```python
from build123d import *
from build123d.topology import SkipClean

# Parameters (mm, degrees)
SKETCH1_W               = 29
SKETCH1_H               = 50
BOSS_EXTRUDE1_DEPTH     = 2.5
SKETCH2_R               = 14.5
SKETCH2_R_2             = 13.8
BOSS_EXTRUDE3_DEPTH     = 6
BOSS_EXTRUDE4_DEPTH     = 6
CUT_EXTRUDE1_DEPTH      = 6
SKETCH5_R               = 0.6
CUT_EXTRUDE2_DEPTH      = 6
CUT_EXTRUDE3_DEPTH      = 10
CUT_EXTRUDE3_DEPTH_BACK = 4
SKETCH6_R               = 1.6
BOSS_EXTRUDE6_DEPTH     = 4
CUT_EXTRUDE4_START      = -8
CUT_EXTRUDE4_DEPTH      = 8
CUT_EXTRUDE5_DEPTH      = 5
SKETCH10_W              = 4.15
SKETCH10_H              = 4.15
SKETCH10_R              = 12.5
CUT_EXTRUDE7_DEPTH      = 1
SKETCH11_W              = 4.15
SKETCH11_H              = 4.15
BOSS_EXTRUDE7_DEPTH     = 2
SKETCH13_R              = 1.1
CUT_EXTRUDE8_DEPTH      = 1.1
SKETCH14_R              = 12.5
CUT_EXTRUDE9_DEPTH      = 1
SKETCH15_R              = 13.8
BOSS_EXTRUDE8_DEPTH     = 0.5
SKETCH16_R              = 14.5
SKETCH16_R_2            = 13.8
BOSS_EXTRUDE9_DEPTH     = 0.5


with BuildPart() as part:
    # Sketch1 → Boss-Extrude1 (new body)
    with BuildSketch(Plane(origin=(0, 0, 0), x_dir=(1, 0, 0), z_dir=(0, 1, 0))):
        with Locations((-98.70287726, -30.536357795)):
            Rectangle(SKETCH1_W, SKETCH1_H)
    extrude(amount=BOSS_EXTRUDE1_DEPTH)

    # Sketch2 → Boss-Extrude3 (add)
    with BuildSketch(Plane(origin=(0, 2.5, 0), x_dir=(1, 0, 0), z_dir=(0, 1, 0))):
        with Locations(Location((-98.70287726, -41.036357795, 0), (0, 0, 270))):
            Circle(SKETCH2_R)
        with Locations(Location((-98.70287726, -41.036357795, 0), (0, 0, 270))):
            Circle(SKETCH2_R_2, mode=Mode.SUBTRACT)
    extrude(amount=BOSS_EXTRUDE3_DEPTH)

    # Sketch3 → Boss-Extrude4 (add)
    with BuildSketch(Plane(origin=(0, 2.5, 0), x_dir=(1, 0, 0), z_dir=(0, 1, 0))):
        with BuildLine():
            Line((-100.672014126, -40.686357795), (-98.70287726, -40.686357795))
            Line((-98.70287726, -40.686357795), (-96.733740393, -40.686357795))
            ThreePointArc((-96.733740393, -40.686357795), (-98.70287726, -39.036357795), (-100.672014126, -40.686357795))
        make_face()
        with BuildLine():
            Line((-96.733740393, -41.386357795), (-100.672014126, -41.386357795))
            ThreePointArc((-100.672014126, -41.386357795), (-98.70287726, -43.036357795), (-96.733740393, -41.386357795))
        make_face()
    extrude(amount=BOSS_EXTRUDE4_DEPTH)

    # Sketch4 → Cut-Extrude1 (cut)
    with BuildSketch(Plane(origin=(0, 2.5, 0), x_dir=(1, 0, 0), z_dir=(0, 1, 0))):
        Polygon((-93.70287726, -26.248512358), (-93.70287726, -14.248512358), (-97.70287726, -14.248512358), (-97.70287726, -20.248512358), (-97.70287726, -26.248512358), align=None)
    extrude(amount=-CUT_EXTRUDE1_DEPTH, mode=Mode.SUBTRACT)

    # Sketch5 → Cut-Extrude2 (cut)
    with BuildSketch(Plane(origin=(0, 0, 26.248512358), x_dir=(-1, 0, 0), z_dir=(0, 0, -1))):
        with Locations((95.70287726, 6)):
            Circle(SKETCH5_R)
    extrude(amount=-CUT_EXTRUDE2_DEPTH, mode=Mode.SUBTRACT)

    # Sketch6 → Cut-Extrude3 (cut, two sides: drawn at the far end of the back side and taken through both)
    with BuildSketch(Plane(origin=(-97.70287726, 0, 0), x_dir=(0, 0, -1), z_dir=(1, 0, 0)).offset(-CUT_EXTRUDE3_DEPTH_BACK)):
        with Locations((-20.248512358, 2.5)):
            Circle(SKETCH6_R)
    extrude(amount=CUT_EXTRUDE3_DEPTH + CUT_EXTRUDE3_DEPTH_BACK, mode=Mode.SUBTRACT)

    # Sketch7 → Boss-Extrude6 (add)
    with SkipClean():  # the faces are left unmerged after this step: merging them gives an invalid solid
        with BuildSketch(Plane(origin=(-97.70287726, 0, 0), x_dir=(0, 0, -1), z_dir=(1, 0, 0))):
            with BuildLine():
                Line((-22.748512358, 2.5), (-21.848512358, 2.5))
                ThreePointArc((-21.848512358, 2.5), (-20.248512358, 4.1), (-18.648512358, 2.5))
                Line((-18.648512358, 2.5), (-17.748512358, 2.5))
                ThreePointArc((-17.748512358, 2.5), (-20.248512358, 5), (-22.748512358, 2.5))
            make_face()
            with BuildLine():
                ThreePointArc((-18.648512358, 2.5), (-20.248512358, 0.9), (-21.848512358, 2.5))
                Line((-21.848512358, 2.5), (-22.748512358, 2.5))
                ThreePointArc((-22.748512358, 2.5), (-20.248512358, 0), (-17.748512358, 2.5))
                Line((-17.748512358, 2.5), (-18.648512358, 2.5))
            make_face()
        extrude(amount=-BOSS_EXTRUDE6_DEPTH)

    # Sketch8 → Cut-Extrude4 (cut)
    with SkipClean():  # the faces are left unmerged after this step: merging them gives an invalid solid
        with BuildSketch(Plane.ZY.offset(93.70287726).offset(CUT_EXTRUDE4_START)):
            with BuildLine():
                Line((20.248512358, 2.5), (18.648512358, 2.5))
                ThreePointArc((18.648512358, 2.5), (19.117141508, 1.36862915), (20.248512358, 0.9))
                Line((20.248512358, 0.9), (20.248512358, 2.5))
            make_face()
            with BuildLine():
                Line((21.848512358, 2.5), (20.248512358, 2.5))
                Line((20.248512358, 2.5), (20.248512358, 0.9))
                ThreePointArc((20.248512358, 0.9), (21.379883208, 1.36862915), (21.848512358, 2.5))
            make_face()
            with BuildLine():
                ThreePointArc((20.248512358, 0.9), (19.117141508, 1.36862915), (18.648512358, 2.5))
                Line((18.648512358, 2.5), (18.648512358, 0.9))
                Line((18.648512358, 0.9), (20.248512358, 0.9))
            make_face()
            with BuildLine():
                ThreePointArc((21.848512358, 2.5), (21.379883208, 1.36862915), (20.248512358, 0.9))
                Line((20.248512358, 0.9), (21.848512358, 0.9))
                Line((21.848512358, 0.9), (21.848512358, 2.5))
            make_face()
        extrude(amount=CUT_EXTRUDE4_DEPTH, mode=Mode.SUBTRACT)

    # Sketch9 → Cut-Extrude5 (cut)
    with SkipClean():  # the faces are left unmerged after this step: merging them gives an invalid solid
        with BuildSketch(Plane(origin=(0, 2.5, 0), x_dir=(1, 0, 0), z_dir=(0, 1, 0))):
            Polygon((-113.20287726, -5.536357795), (-113.20287726, -16.036357795), (-97.70287726, -16.036357795), (-97.70287726, -14.248512358), (-93.70287726, -14.248512358), (-93.70287726, -16.036357795), (-84.20287726, -16.036357795), (-84.20287726, -5.536357795), align=None)
        extrude(amount=-CUT_EXTRUDE5_DEPTH, mode=Mode.SUBTRACT)

    # Sketch10 → Cut-Extrude7 (cut)
    with SkipClean():  # the faces are left unmerged after this step: merging them gives an invalid solid
        with BuildSketch(Plane.XZ):
            with Locations((-111.12787726, 18.111357795)):
                Rectangle(SKETCH10_W, SKETCH10_H)
            with Locations((-86.27787726, 18.111357795)):
                Rectangle(SKETCH10_W, SKETCH10_H)
            with Locations((-111.12787726, 53.461357795)):
                Rectangle(SKETCH10_W, SKETCH10_H)
            with Locations((-86.27787726, 53.461357795)):
                Rectangle(SKETCH10_W, SKETCH10_H)
            with Locations(Location((-98.70287726, 41.036357795, 0), (0, 0, 270))):
                Circle(SKETCH10_R)
        extrude(amount=-CUT_EXTRUDE7_DEPTH, mode=Mode.SUBTRACT)

    # Sketch11 → Boss-Extrude7 (add)
    with SkipClean():  # the faces are left unmerged after this step: merging them gives an invalid solid
        with BuildSketch(Plane(origin=(0, 2.5, 0), x_dir=(1, 0, 0), z_dir=(0, 1, 0))):
            with Locations((-111.12787726, -53.461357795)):
                Rectangle(SKETCH11_W, SKETCH11_H)
            with Locations((-86.27787726, -53.461357795)):
                Rectangle(SKETCH11_W, SKETCH11_H)
            with Locations((-111.12787726, -18.111357795)):
                Rectangle(SKETCH11_W, SKETCH11_H)
            Polygon((-88.35287726, -16.036357795), (-88.35287726, -18.648512358), (-85.70287726, -18.648512358), (-85.70287726, -20.186357795), (-84.20287726, -20.186357795), (-84.20287726, -16.036357795), align=None)
        extrude(amount=BOSS_EXTRUDE7_DEPTH)

    # Sketch13 → Cut-Extrude8 (cut)
    with SkipClean():  # the faces are left unmerged after this step: merging them gives an invalid solid
        with BuildSketch(Plane.XZ.offset(-1)):
            with Locations(Location((-111.12787726, 53.461357795, 0), (0, 0, 270))):
                Circle(SKETCH13_R)
            with Locations(Location((-86.27787726, 53.461357795, 0), (0, 0, 270))):
                Circle(SKETCH13_R)
            with Locations(Location((-111.12787726, 18.111357795, 0), (0, 0, 270))):
                Circle(SKETCH13_R)
            with Locations((-86.27787726, 18.111357795)):
                Circle(SKETCH13_R)
        extrude(amount=-CUT_EXTRUDE8_DEPTH, mode=Mode.SUBTRACT)

    # Sketch14 → Cut-Extrude9 (cut)
    with SkipClean():  # the faces are left unmerged after this step: merging them gives an invalid solid
        with BuildSketch(Plane.XZ.offset(-1)):
            with Locations(Location((-98.70287726, 41.036357795, 0), (0, 0, 270))):
                Circle(SKETCH14_R)
        extrude(amount=-CUT_EXTRUDE9_DEPTH, mode=Mode.SUBTRACT)

    # Sketch15 → Boss-Extrude8 (add)
    with SkipClean():  # the faces are left unmerged after this step: merging them gives an invalid solid
        with BuildSketch(Plane(origin=(0, 2.5, 0), x_dir=(1, 0, 0), z_dir=(0, 1, 0))):
            with Locations(Location((-98.70287726, -41.036357795, 0), (0, 0, 270))):
                Circle(SKETCH15_R)
        extrude(amount=BOSS_EXTRUDE8_DEPTH)

    # Sketch16 → Boss-Extrude9 (add)
    # profile 1 of 3: a face of its own
    with SkipClean():  # the faces are left unmerged after this step: merging them gives an invalid solid
        with BuildSketch(Plane(origin=(0, 8.5, 0), x_dir=(1, 0, 0), z_dir=(0, 1, 0))):
            with Locations(Location((-98.70287726, -41.036357795, 0), (0, 0, 270))):
                Circle(SKETCH16_R)
            with Locations(Location((-98.70287726, -41.036357795, 0), (0, 0, 270))):
                Circle(SKETCH16_R_2, mode=Mode.SUBTRACT)
        # profile 2 of 3: a face of its own
        with BuildSketch(Plane(origin=(0, 8.5, 0), x_dir=(1, 0, 0), z_dir=(0, 1, 0))):
            with BuildLine():
                ThreePointArc((-96.733740393, -40.686357795), (-98.70287726, -39.036357795), (-100.672014126, -40.686357795))
                Line((-100.672014126, -40.686357795), (-96.733740393, -40.686357795))
            make_face()
        # profile 3 of 3: a face of its own
        with BuildSketch(Plane(origin=(0, 8.5, 0), x_dir=(1, 0, 0), z_dir=(0, 1, 0))):
            with BuildLine():
                ThreePointArc((-100.672014126, -41.386357795), (-98.70287726, -43.036357795), (-96.733740393, -41.386357795))
                Line((-96.733740393, -41.386357795), (-100.672014126, -41.386357795))
            make_face()
        extrude(amount=BOSS_EXTRUDE9_DEPTH)


solid = part.part
```
The model under review builds one solid part; all positions refer to its coordinate system, in mm. A direction names the side the tool comes from. Round coordinates to 2 decimals unless told otherwise and drop trailing zeros. Loops run counter-clockwise (first coordinate to the right, second up) from the corner with the lowest first, then second, coordinate; pieces in that order, holes last. Notation, with made-up numbers: (9, -22.5) -> (61, -22.5) arc R35 ccw to (61, 12.5) -> close; hole circle Ø3 at (18, -23.75). An arc over 180 degrees is marked (long way). Answer in a Markdown table with one row per item.
1) Tool access review of faces 1 (the cylindrical face through (-98.742, 5.958, 43.036)), 2 (the flat face through (-86, 4.5, 18)), 3 (the flat face through (-111, 3, 51.386)), 4 (the cylindrical face through (-86.035, 1.542, 17.038)): name each direction out of +Z, -Z, +X, -X, +Y, -Y from which nothing blocks a thin tool from reaching the whole face with its end or side.
Taken from the geometry:
| item | result |
|---|---|
| face 1 | +Y |
| face 2 | -Z, +X, +Y |
| face 3 | -X, +Y |
| face 4 | -Y |
2) For pin 1 Ø2 at (x, y) = (-95, 1.5) entering from -Z; pin 2 Ø2 at (x, z) = (-111.13, 53.46) entering from -Y; pin 3 Ø3 at (x, y) = (-91.5, 4.5) entering from -Z, all flat-tipped, find the tip position at first contact; note any pin that passes through.
Taken from the geometry:
| item | result |
|---|---|
| pin 1 | stops at z = 26.25 |
| pin 2 | stops at y = 2.1 |
| pin 3 | stops at z = 27.7 |
3) Consider section D-D, the plane z = 47. Write out the cut boundary in (x, y), plus the area to 3 significant figures.
Taken from the geometry:
| item | result |
|---|---|
| outline | (-113.2, 0) -> (-109.69, 0) -> (-109.69, 2) -> (-87.72, 2) -> (-87.72, 0) -> (-84.2, 0) -> (-84.2, 2.5) -> (-85.49, 2.5) -> (-85.49, 9) -> (-86.26, 9) -> (-86.26, 3) -> (-111.15, 3) -> (-111.15, 9) -> (-111.92, 9) -> (-111.92, 2.5) -> (-113.2, 2.5) -> close |
| area | 51.0 mm² |
4) Wall thickness on line 1 along Z through (x, y) = (-109.75, 3.75); line 2 along X through (y, z) = (7.75, 40); line 3 along X through (y, z) = (8, 40.5): over which ranges is each line inside the solid? List them lowest first.
Taken from the geometry:
| item | result |
|---|---|
| line 1 | z = 16.04 to 20.19, 31.64 to 32.77, 49.31 to 50.43, 51.39 to 55.54 |
| line 2 | x = -113.17 to -112.46, -100.41 to -96.99, -84.94 to -84.24 |
| line 3 | x = -113.19 to -112.49, -100.63 to -96.78, -84.91 to -84.21 |
5) Consider section C-C, the plane y = 6. Write out the cut boundary in (x, z), plus the area to 3 significant figures.
Taken from the geometry:
| item | result |
|---|---|
| outline | (-100.67, 40.69) arc R2 ccw to (-96.73, 40.69) -> close; (-100.67, 41.39) -> (-96.73, 41.39) arc R2 ccw to start; (-96.3, 26.74) -> (-96.3, 27.45) arc R13.8 cw (long way) to (-95.1, 27.71) -> (-95.1, 26.99) arc R14.5 ccw (long way) to start |
| area | 71.2 mm² |
6) Consider section B-B, the plane y = 8.5. Write out the cut boundary in (x, z).
Taken from the geometry:
| item | result |
|---|---|
| outline | circle Ø29 at (-98.7, 41.04); (-100.67, 40.69) arc R2 ccw to (-96.73, 40.69) -> close; (-100.67, 41.39) -> (-96.73, 41.39) arc R2 ccw to start; hole circle Ø27.6 at (-98.7, 41.04) |
7) Consider section A-A, the plane y = 3.5. Count the separate pieces of the cut face and the enclosed holes in it, plus the area to 3 significant figures.
Taken from the geometry:
| item | result |
|---|---|
| separate pieces | 9 |
| enclosed holes | 1 |
| area | 145 mm² |
8) Draft analysis for pull direction Z (two halves, no side actions). For faces 5 (the cylindrical face through (-98.664, 5.958, 39.037)), 6 (the flat face through (-84.203, 2, 36)), 7 (the flat face through (-96, 1, 26.249)), 8 (the cylindrical face through (-99.7, 5, 20.2)), state which applies: pulls with the +Z half, pulls with the -Z half, needs draft (parallel to the pull), parting line crosses it, or undercut.
Taken from the geometry:
| item | result |
|---|---|
| face 5 | undercut |
| face 6 | needs draft |
| face 7 | pulls with the -Z half |
| face 8 | undercut |
